Autodesk Inventor part; units mm, degrees
ref_plane "Work Plane1" through (1.525, 0, 0) normal (0, 0, 1) x (1, 0, 0)
ref_plane "YZ Plane" through (0, 0, 0) normal (1, 0, 0) x (0, 1, 0)
ref_plane "XZ Plane" through (0, 0, 0) normal (0, 1, 0) x (-1, 0, 0)
sketch "Skizze1" plane through (0, 0, 0) normal (0, 0, 1) x (1, 0, 0)
  line L0 (0, 3.45) -> (0, 2.5)
  line L1 (9, 2.5) -> (25, 2.5)
  line L2 (25, 2.5) -> (25, 0)
  line L3 (25, 0) -> (-0.5001, 0)
  line L4 (-5.6001, 0) -> (30.1, 0)
  line L5 (-0.5001, 0) -> (-0.5001, 3.45)
  line L6 (-0.5001, 3.45) -> (0, 3.45)
  line L7 (9, 2.5) -> (8.5091, 2.5)
  line L8 (8.5091, 2.5) -> (0, 2.5)
  line L9 (0, -0.69) -> (0, 4.14)
  dimension "d0" = 25
  dimension "d1" = 16
  dimension "d2" = 5
  dimension "d9" = 0.5001
  dimension "d10" = 6.9
  dimension "d13" = 0.4909
  dimension "d14" = 5
revolve "Körper" add sketch "Skizze1" angle 360 about axis through (25, 0, 0) along (-1, 0, 0)
sketch "Skizze2" plane through (-0.5001, 0, 0) normal (-1, 0, 0) x (0, 0, 1)
  line L0 (0, 4.6188) -> (4, 2.3094)
  line L1 (4, 2.3094) -> (4, -2.3094)
  line L2 (4, -2.3094) -> (0, -4.6188)
  line L3 (0, -4.6188) -> (-4, -2.3094)
  line L4 (-4, -2.3094) -> (-4, 2.3094)
  line L5 (-4, 2.3094) -> (0, 4.6188)
  point P0 (0, 0)
  point P1 (0, 0)
  dimension "d11" = 8
extrude "Kopf" add sketch "Skizze2" along normal blind 3
sketch "Skizze4" plane through (0, 0, 0) normal (0, 0, 1) x (1, 0, 0)
  line L0 (-3.5001, 4) -> (-3.5001, 4.6188)
  line L1 (-3.5001, 4.6188) -> (-3.1428, 4.6188)
  line L2 (-3.1428, 4.6188) -> (-3.5001, 4)
  line L3 (-4.1001, 0) -> (0.0999, 0)
  line L4 (-0.5001, 4.6188) -> (-3.5001, 4.6188)
  line L5 (-3.5001, 2.3094) -> (-3.5001, 4.6188)
  dimension "d5" = 30
  dimension "d19" = 8
revolve "Fase1" cut sketch "Skizze4" angle 360 about axis through (-10, 0, 0) along (1, 0, 0)
thread "Gewinde"
chamfer "Fase2" distance 0.4908 distance2 0.4909 1 edges at (25, -2.5, 0) measured on face at (25, 0.7379, -0.3873)
ref_plane "Work Plane1" through (1.525, 0, 0) normal (0, 0, 1) x (1, 0, 0)
equation "\"d0\" = NLG"
equation "\"d1\" = GEL"
equation "\"d2\" = GD"
equation "\"d10\" = SD2"
equation "\"d14\" = BDM"
equation "\"d11\" = SW"
equation "\"d3\" = KOH - SD"
equation "\"d5\" = ANG1"
equation "\"d19\" = SW0"
equation "\"d15\" = GEL"
equation "\"d6\" = -0.5 * SPD + 0.5 * GD"
equation "\"NLG\" = 25"
equation "\"GD\" = NND"
equation "\"BDM\" = NND"
equation "\"KOH\" = 3.5"
equation "\"GEL\" = 16"
equation "\"SW\" = 8"
equation "\"SW0\" = SW"
equation "\"SPD\" = NND - 1.2269 * PTC"
equation "\"SD2\" = 6.9"
equation "\"SD\" = 0.5"
equation "\"ANG1\" = 30deg"
equation "\"GAL\" = 0.61345 * PTC"
equation "\"GUL\" = 0.61345 * PTC"
equation "\"RR\" = 0.2"
equation "\"GD1\" = THREADDIA - 1.2269 * PTC"
equation "\"THREADDIA\" = 5"
equation "\"TOA\" = 30deg"
equation "\"PTC\" = 0.8"
equation "\"NND\" = 5"
equation "\"E0\" = 1.155 * SW"
properties part number "DIN 931-1 - M5 x 25" material "Stahl, weich"
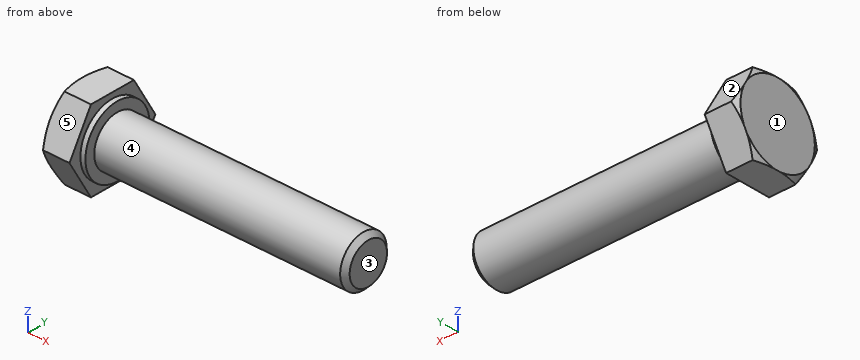
Build history of the part. All positions in model axes, mm. Face numbers are marked on the shaded views. A direction names the side the tool comes from. Round coordinates to 2 decimals unless told otherwise and drop trailing zeros. Write each loop counter-clockwise with the first axis right and the second up, starting at its lowest first coordinate (ties: lowest second). Pieces come first, ordered by that corner, then holes. Notation, with made-up numbers: (77, -36) - (120, -36) arc R29 ccw to (120, -12) - close; hole circle Ø11 at (79, 64.5). An arc over 180 degrees is marked (long way). Use CSV: the item, a comma, the result in double quotes.
(1) 3-axis set-ups, long thin cutter, end or side, ignore diameter. For the marked faces 4 and 5: which of +Z, -Z, +X, -X, +Y, -Y reach the whole face in a straight line?
Response:
face 4,"+X"
face 5,"+Z, +X, -X, -Y"
(2) Mould opens along X. For the marked faces 1, 2 and 3 say: pulls with the +X half, pulls with the -X half, needs draft (parallel to the pull), parting line crosses it, or undercut.
Response:
face 1,"pulls with the -X half"
face 2,"needs draft"
face 3,"pulls with the +X half"
(3) Wall check: line 1 (Y direction, x = 15.5, z = 1.5); line 2 (X direction, y = -3, z = 0.25); line 3 (Z direction, x = 23.5, y = 0). Give the ranges that are in metal, low to high.
Response:
line 1,"-2 to 2"
line 2,"-3.5 to 0"
line 3,"-2.5 to 2.5"
(4) Pin check, flat tips, straight feed: P1, Ø5, axis at x = 18.5, y = -1, coming from the +Z side; P2, Ø1.5, axis at y = -2.5, z = -1.5, coming from the +X side. Stop position of each tip, or through.
Response:
P1,"z = 2.5"
P2,"x = 24.84"
(5) Band-saw the part on A-A (x = 22.75). Write the cut outline in (y, z), plus the area to 3 significant figures.
Response:
outline,"circle Ø5 at (0, 0)"
area,"19.6 mm²"
